Check sheet for the modelled part. Datum: model origin and axes. Units: mm. A direction names the side the tool comes from. Round coordinates to 2 decimals unless told otherwise and drop trailing zeros. Write each loop counter-clockwise with the first axis right and the second up, starting at its lowest first coordinate (ties: lowest second). Pieces come first, ordered by that corner, then holes.
Item 1: Cross-section at A-A on z = 0. Count the separate pieces of the cut face and the enclosed holes in it, plus the area to 3 significant figures.
Item 2: Tool access check on faces 1 (the cylindrical face through (4.366, -10.488, 0.108)), 2 (the cylindrical face through (2, 5, 0)), 3 (the cylindrical face through (3, -5, 0)). Record the directions out of +Z, -Z, +X, -X, +Y, -Y that give a thin tool (end or side, any length) a straight path to the whole face; none if there is none.
Item 3: Cross-section at B-B on y = -2. Enter the section's corners in (x, z).
Item 4: Release check for a two-part mould opening along Y. For faces 4 (the cylindrical face through (0.616, -10.488, 0.108)), 5 (the cylindrical face through (0.6, 11.5, 0)), 6 (the cylindrical face through (2.465, -3.265, -3.332)) record: +Y half, -Y half, draft (parallel to the pull), parting line (faces both ways), or undercut.
Item 5: Cross-section at D-D on y = -6.25. Enter the section's corners in (x, z), plus the area to 3 significant figures.
Item 6: Material ranges on line 1 (Y direction, x = 4.4, z = 0); line 2 (X direction, y = -7, z = -1.25); line 3 (Y direction, x = 1.9, z = 0), recorded low to high.
Item 7: Go/stop test with flat-tipped pins: pin 1 Ø3 at (x, y) = (3.5, 3.5) entering from +Z; pin 2 Ø1 at (x, y) = (3.5, 3) entering from -Z; pin 3 Ø1.5 at (x, y) = (4.5, 4) entering from -Z. Record where each tip stops, or that it passes through.
from build123d import *

# Parameters (mm, degrees)
CROQUIS1_R              = 2.5
CROQUIS1_R_2            = 0.5
SALIENTE_EXTRUIR1_DEPTH = 5
REDONDEO1_R             = 50
REDONDEO2_R             = 10
CORTAR_EXTRUIR1_START   = -2.5
CORTAR_EXTRUIR1_DEPTH   = 1.25


with BuildPart() as part:
    # Croquis1 → Saliente-Extruir1 (new body)
    with BuildSketch(Plane(origin=(0, 0, 0), x_dir=(0, 0, -1), z_dir=(1, 0, 0))):
        with BuildLine():
            ThreePointArc((-1.5, -10), (0, -11.5), (1.5, -10))
            ThreePointArc((1.5, -10), (2.97123258, -5.077902331), (3.75, 0))
            ThreePointArc((3.75, 0), (2.97123258, 5.077902331), (1.5, 10))
            ThreePointArc((1.5, 10), (0, 11.5), (-1.5, 10))
            ThreePointArc((-1.5, 10), (-2.97123258, 5.077902331), (-3.75, 0))
            ThreePointArc((-3.75, 0), (-2.97123258, -5.077902331), (-1.5, -10))
        make_face()
        Circle(CROQUIS1_R, mode=Mode.SUBTRACT)
        with Locations((0, 10)):
            Circle(CROQUIS1_R_2, mode=Mode.SUBTRACT)
        with Locations((0, -10)):
            Circle(CROQUIS1_R_2, mode=Mode.SUBTRACT)
    extrude(amount=SALIENTE_EXTRUIR1_DEPTH)

    # Redondeo1
    redondeo1_edges = [part.edges().sort_by_distance(p)[0] for p in [
        (2.5, 10, 1.5),
        (2.5, 10, -1.5),
        (2.5, -10, -1.5),
        (2.5, -10, 1.5),
    ]]
    fillet(redondeo1_edges, radius=REDONDEO1_R)

    # Redondeo2
    redondeo2_edges = [part.edges().sort_by_distance(p)[0] for p in [
        (2.5, 0, -3.75),
        (2.5, 0, 3.75),
    ]]
    fillet(redondeo2_edges, radius=REDONDEO2_R)

    # Croquis2 → Cortar-Extruir1 (cut, symmetric)
    with BuildSketch(Plane.ZY.offset(CORTAR_EXTRUIR1_START)):
        with BuildLine():
            ThreePointArc((-3.232551289, -3.814526467), (0, -5), (3.232551289, -3.814526467))
            ThreePointArc((3.232551289, -3.814526467), (2.705759395, -6.179171669), (2.02610144, -8.504493518))
            ThreePointArc((2.02610144, -8.504493518), (1.724946708, -9.454502859), (1.442786447, -10.410325806))
            ThreePointArc((1.442786447, -10.410325806), (0, -11.5), (-1.442786447, -10.410325806))
            ThreePointArc((-1.442786447, -10.410325806), (-1.724946708, -9.454502859), (-2.02610144, -8.504493518))
            ThreePointArc((-2.02610144, -8.504493518), (-2.705759395, -6.179171669), (-3.232551289, -3.814526467))
        make_face()
        with BuildLine():
            ThreePointArc((3.232551289, 3.814526467), (0, 5), (-3.232551289, 3.814526467))
            ThreePointArc((-3.232551289, 3.814526467), (-2.705759395, 6.179171669), (-2.02610144, 8.504493518))
            ThreePointArc((-2.02610144, 8.504493518), (-1.724946708, 9.454502859), (-1.442786447, 10.410325806))
            ThreePointArc((-1.442786447, 10.410325806), (0, 11.5), (1.442786447, 10.410325806))
            ThreePointArc((1.442786447, 10.410325806), (1.724946708, 9.454502859), (2.02610144, 8.504493518))
            ThreePointArc((2.02610144, 8.504493518), (2.705759395, 6.179171669), (3.232551289, 3.814526467))
        make_face()
    extrude(amount=CORTAR_EXTRUIR1_DEPTH, both=True, mode=Mode.SUBTRACT)


solid = part.part
Response values:
1. separate pieces: 6
1. enclosed holes: 0
1. area: 52.5 mm2
2. face 1: +X, -X
2. face 2: +Y
2. face 3: -Y
3. outline: (0, -3.53) - (5, -3.53) - (5, -1.5) - (0, -1.5) - close; (0, 1.5) - (5, 1.5) - (5, 3.53) - (0, 3.53) - close
4. face 4: undercut
4. face 5: +Y half
4. face 6: -Y half
5. outline: (0, -2.69) - (1.25, -2.69) - (1.25, 2.69) - (0, 2.69) - close; (3.75, -2.69) - (5, -2.69) - (5, 2.69) - (3.75, 2.69) - close
5. area: 13.4 mm2
6. line 1: y = -11.5 to -10.5, -9.5 to -2.5, 2.5 to 9.5, 10.5 to 11.5
6. line 2: x = 0 to 1.25, 3.75 to 5
6. line 3: y = -5 to -2.5, 2.5 to 5
7. pin 1: stops at z = 3.53
7. pin 2: stops at z = -3.46
7. pin 3: stops at z = -3.33
